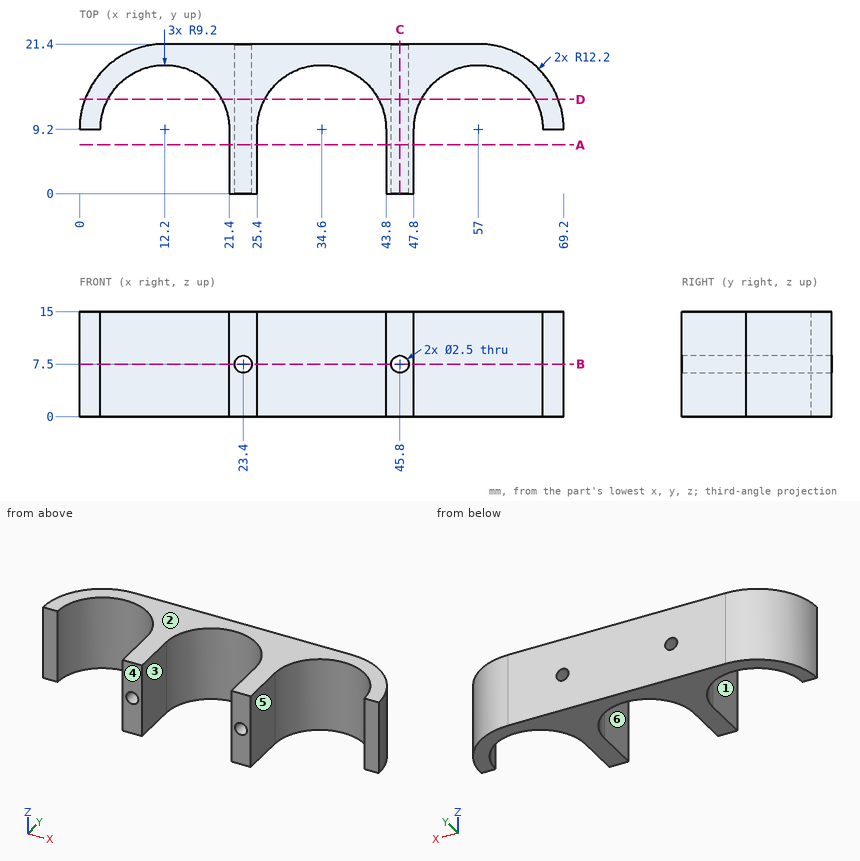
The figure shows three views and two pictorial views of one solid part (mm, origin at its lowest corner). Answer the questions. A direction names the side the tool comes from. Round coordinates to 2 decimals unless told otherwise and drop trailing zeros. Order: outer loops, then holes, each group sorted by start corner. A loop starts at its lowest first (then second) coordinate and runs counter-clockwise, first axis right, second up.
Q1. The mould has two halves that part along X. Classify the marked faces 1, 2 and 3: pulls with the +X half, pulls with the -X half, needs draft (parallel to the pull), parting line crosses it, or undercut.
Solution:
face 1: pulls with the -X half
face 2: needs draft
face 3: undercut
Q2. A cutting plane is placed at A-A, the plane y = 7. Determine the outline of the cut face in (x, z).
Solution:
outline: (21.4, 0) - (25.4, 0) - (25.4, 15) - (21.4, 15) - close; (43.8, 0) - (47.8, 0) - (47.8, 15) - (43.8, 15) - close; hole circle Ø2.5 at (23.4, 7.5); hole circle Ø2.5 at (45.8, 7.5)
Q3. A cutting plane is placed at C-C, the plane x = 45.8. Determine the outline of the cut face in (y, z), then the cut area to 4 significant figures.
Solution:
outline: (0, 0) - (21.4, 0) - (21.4, 6.25) - (0, 6.25) - close; (0, 8.75) - (21.4, 8.75) - (21.4, 15) - (0, 15) - close
area: 267.5 mm2
Q4. Find the intervals of material crossed by line 1 along X through (y, z) = (9.5, 7.5); line 2 along Z through (x, y) = (45.8, 5); line 3 along X through (y, z) = (15.75, 14), in increasing order.
Solution:
line 1: x = 0 to 3, 21.4 to 22.15, 24.65 to 25.4, 43.8 to 44.55, 47.05 to 47.8, 66.2 to 69.2
line 2: z = 0 to 6.25, 8.75 to 15
line 3: x = 1.91 to 5.74, 18.66 to 28.14, 41.06 to 50.54, 63.46 to 67.29
Q5. A cutting plane is placed at D-D, the plane y = 13.5. Determine the outline of the cut face in (x, z), then the cut area to 3 significant figures.
Solution:
outline: (0.78, 0) - (4.07, 0) - (4.07, 15) - (0.78, 15) - close; (20.33, 0) - (26.47, 0) - (26.47, 15) - (20.33, 15) - close; (42.73, 0) - (48.87, 0) - (48.87, 15) - (42.73, 15) - close; (65.13, 0) - (68.42, 0) - (68.42, 15) - (65.13, 15) - close; hole circle Ø2.5 at (23.4, 7.5); hole circle Ø2.5 at (45.8, 7.5)
area: 273 mm2
Q6. Given pin 1 Ø6 at (y, z) = (12.5, 5) entering from -X; pin 2 Ø3 at (y, z) = (4.5, 4) entering from +X; pin 3 Ø2.5 at (x, z) = (67, 5) entering from -Y; pin 4 Ø2 at (x, z) = (45.8, 7.5) entering from -Y, each flat-ended and moving along its own axis, determine where each tip first touches the part or whether it passes through.
Solution:
pin 1: stops at x = 0
pin 2: stops at x = 47.8
pin 3: stops at y = 9.2
pin 4: passes through
Q7. A tool of negligible diameter and unlimited length cuts with its end or side. For the marked faces 4, 5 and 6, from which of +Z, -Z, +X, -X, +Y, -Y can it reach the whole face along a straight path? Write none if from no direction.
Solution:
face 4: +Z, -Z, +X, -X, -Y
face 5: +Z, -Z, +X, -Y
face 6: +Z, -Z, -Y
Q8. A cutting plane is placed at B-B, the plane z = 7.5. Determine the outline of the cut face in (x, y).
Solution:
outline: (0, 9.2) - (3, 9.2) arc R9.2 cw to (21.4, 9.2) - (21.4, 0) - (22.15, 0) - (22.15, 21.4) - (12.2, 21.4) arc R12.2 ccw to start; (24.65, 0) - (25.4, 0) - (25.4, 9.2) arc R9.2 cw to (43.8, 9.2) - (43.8, 0) - (44.55, 0) - (44.55, 21.4) - (24.65, 21.4) - close; (47.05, 0) - (47.8, 0) - (47.8, 9.2) arc R9.2 cw to (66.2, 9.2) - (69.2, 9.2) arc R12.2 ccw to (57, 21.4) - (47.05, 21.4) - close
